Geometry check sheet. Reference: drawing and pictorial views, mm from the part's lowest x, y, z. A direction names the side the tool comes from. Coordinates: 2 decimals unless noted, no trailing zeros. Write each loop counter-clockwise with the first axis right and the second up, starting at its lowest first coordinate (ties: lowest second). Pieces come first, ordered by that corner, then holes. Notation, with made-up numbers: (71.25, 28) -> (122.25, 28) arc R26 ccw to (122.25, 66) -> close; hole circle Ø1 at (-19.75, 10). An arc over 180 degrees is marked (long way). Answer in a Markdown table with one row per item.
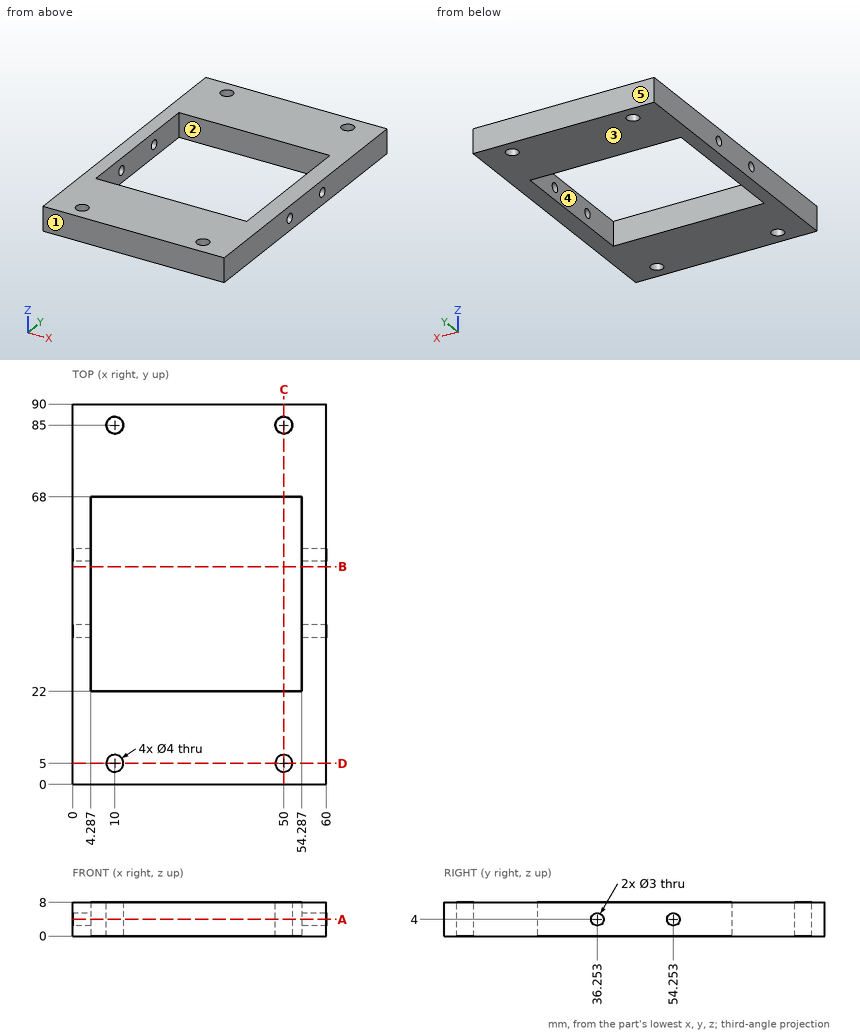
1. Section check B-B, the plane y = 51.5. Record the boundary of the cut face in (x, z).
Geometry says:
| item | result |
|---|---|
| outline | (0, 0) -> (4.29, 0) -> (4.29, 8) -> (0, 8) -> close; (54.29, 0) -> (60, 0) -> (60, 8) -> (54.29, 8) -> close |
2. Tool access check on the marked faces 1 and 2. Record the directions out of +Z, -Z, +X, -X, +Y, -Y that give a thin tool (end or side, any length) a straight path to the whole face; none if there is none.
Geometry says:
| item | result |
|---|---|
| face 1 | +Z, -Z, +X, -X, -Y |
| face 2 | +Z, -Z |
3. Mould release check, pull along Y, two halves, no side actions. Record for the marked faces 3, 4 and 5: released by +Y, released by -Y, zero draft, split by the parting line, or undercut.
Geometry says:
| item | result |
|---|---|
| face 3 | zero draft |
| face 4 | undercut |
| face 5 | released by +Y |
4. Thickness scan on line 1 (Y direction, x = 10, z = 4.5); line 2 (X direction, y = 85, z = 6); line 3 (Y direction, x = 57.25, z = 4). Record the ranges inside material, lowest first. Write a range as from..to.
Geometry says:
| item | result |
|---|---|
| line 1 | 0..3, 7..22, 68..83, 87..90 |
| line 2 | 0..8, 12..48, 52..60 |
| line 3 | 0..34.75, 37.75..52.75, 55.75..90 |
5. Section check A-A, the plane z = 4. Record the boundary of the cut face in (x, y).
Geometry says:
| item | result |
|---|---|
| outline | (0, 0) -> (60, 0) -> (60, 34.75) -> (54.29, 34.75) -> (54.29, 22) -> (4.29, 22) -> (4.29, 34.75) -> (0, 34.75) -> close; (0, 37.75) -> (4.29, 37.75) -> (4.29, 52.75) -> (0, 52.75) -> close; (0, 55.75) -> (4.29, 55.75) -> (4.29, 68) -> (54.29, 68) -> (54.29, 55.75) -> (60, 55.75) -> (60, 90) -> (0, 90) -> close; (54.29, 37.75) -> (60, 37.75) -> (60, 52.75) -> (54.29, 52.75) -> close; hole circle Ø4 at (10, 5); hole circle Ø4 at (10, 85); hole circle Ø4 at (50, 5); hole circle Ø4 at (50, 85) |
6. Section check C-C, the plane x = 50. Record the boundary of the cut face in (y, z).
Geometry says:
| item | result |
|---|---|
| outline | (0, 0) -> (3, 0) -> (3, 8) -> (0, 8) -> close; (7, 0) -> (22, 0) -> (22, 8) -> (7, 8) -> close; (68, 0) -> (83, 0) -> (83, 8) -> (68, 8) -> close; (87, 0) -> (90, 0) -> (90, 8) -> (87, 8) -> close |
7. Section check D-D, the plane y = 5. Record the boundary of the cut face in (x, z).
Geometry says:
| item | result |
|---|---|
| outline | (0, 0) -> (8, 0) -> (8, 8) -> (0, 8) -> close; (12, 0) -> (48, 0) -> (48, 8) -> (12, 8) -> close; (52, 0) -> (60, 0) -> (60, 8) -> (52, 8) -> close |
8. Depth check by flat-ended pin: P1, Ø3.5, axis at x = 50, y = 85, coming from the +Z side; P2, Ø2.5, axis at y = 34.5, z = 4.5, coming from the -X side. Enter the tip coordinate at first touch or a pass-through.
Geometry says:
| item | result |
|---|---|
| P1 | through |
| P2 | x = 0 |
